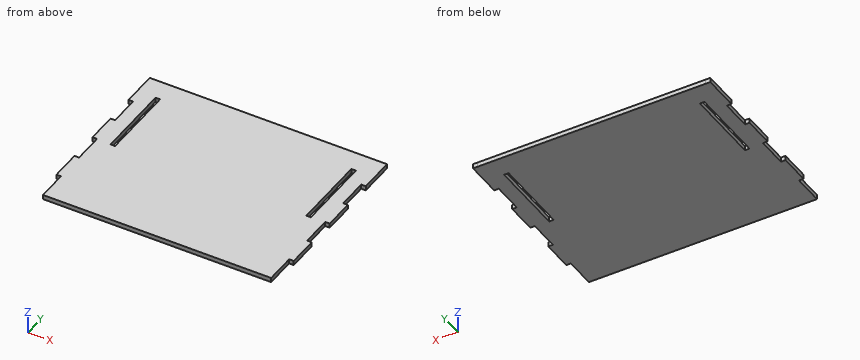
```python
from build123d import *

# Parameters (mm, degrees)
SKETCH1_W           = 6
SKETCH1_H           = 100.000000002
BOSS_EXTRUDE1_DEPTH = 6


with BuildPart() as part:
    # Sketch1 → Boss-Extrude1 (new body)
    with BuildSketch(Plane.XY):
        Polygon((-302, 181.40990873), (-2, 181.409908735), (4, 181.409908735), (4, 134.306809003), (-2, 134.306809003), (-2, 94.306809003), (4, 94.306809003), (4, 54.306809003), (-2, 54.306809003), (-2, 14.306809003), (4, 14.306809003), (4, -25.693190997), (-2, -25.693190997), (-2, -65.693190997), (-302, -65.693190997), (-302, -25.693191002), (-308, -25.693191002), (-308, 14.306808998), (-302, 14.306808998), (-302, 54.306808998), (-308, 54.306808998), (-308, 94.306808998), (-302, 94.306808998), (-302, 134.306808998), (-308, 134.306808998), (-308, 181.40990873), align=None)
        with Locations((-280.75, 103.306809004)):
            Rectangle(SKETCH1_W, SKETCH1_H, mode=Mode.SUBTRACT)
        with Locations((-23.25, 103.306809004)):
            Rectangle(SKETCH1_W, SKETCH1_H, mode=Mode.SUBTRACT)
    extrude(amount=BOSS_EXTRUDE1_DEPTH)


solid = part.part
```
The listing builds one solid part. Answer for the finished solid, in the listing's coordinates (mm). Coordinates: 2 decimals unless noted, no trailing zeros. Loops run counter-clockwise (first coordinate to the right, second up) from the corner with the lowest first, then second, coordinate; pieces in that order, holes last. Notation, with made-up numbers: (62.25, 39) - (87.25, 39) arc R16 ccw to (87.25, 57) - close; hole circle Ø3 at (30.5, -26.5). An arc over 180 degrees is marked (long way). Use a Markdown table: item, result. Add a question column.
1) Given pin 1 (1.8 mm diameter, centred on y = 121, z = 4, fed in from -X); pin 2 (3 mm diameter, centred on y = 29, z = 3.5, fed in from +X), each flat-ended and moving along its own axis, determine where each tip first touches the part or whether it passes through.
2) Find the intervals of material crossed by line 1 (X direction, y = 93, z = 1.2); line 2 (X direction, y = 118, z = 4.55); line 3 (X direction, y = -42, z = 3.2), in increasing order.
3) The part is cut by section C-C, the plane y = 82.5. Give the vertices of the cut face in (x, z).
4) The part is cut by section B-B, the plane z = 4.65. State how many separate pieces and enclosed holes the cut face has, and give its area (3 significant figures).
5) The part is cut by section D-D, the plane y = -38. Give the vertices of the cut face in (x, z), and give its area (3 significant figures).
6) The part is cut by section A-A, the plane y = 129. Give the vertices of the cut face in (x, z).
Here are the results:
| question | item | result |
|---|---|---|
| 1 | pin 1 | stops at x = -302 |
| 1 | pin 2 | stops at x = -2 |
| 2 | line 1 | x = -308 to -283.75, -277.75 to -26.25, -20.25 to 4 |
| 2 | line 2 | x = -302 to -283.75, -277.75 to -26.25, -20.25 to -2 |
| 2 | line 3 | x = -302 to -2 |
| 3 | outline | (-308, 0) - (-283.75, 0) - (-283.75, 6) - (-308, 6) - close; (-277.75, 0) - (-26.25, 0) - (-26.25, 6) - (-277.75, 6) - close; (-20.25, 0) - (4, 0) - (4, 6) - (-20.25, 6) - close |
| 4 | separate pieces | 1 |
| 4 | enclosed holes | 2 |
| 4 | area | 74,500 mm^2 |
| 5 | outline | (-302, 0) - (-2, 0) - (-2, 6) - (-302, 6) - close |
| 5 | area | 1,800 mm^2 |
| 6 | outline | (-302, 0) - (-283.75, 0) - (-283.75, 6) - (-302, 6) - close; (-277.75, 0) - (-26.25, 0) - (-26.25, 6) - (-277.75, 6) - close; (-20.25, 0) - (-2, 0) - (-2, 6) - (-20.25, 6) - close |
